Verification items for the finished model (mm, model axes). Coordinates: 2 decimals unless noted, no trailing zeros. Write each loop counter-clockwise with the first axis right and the second up, starting at its lowest first coordinate (ties: lowest second). Pieces come first, ordered by that corner, then holes. Notation, with made-up numbers: (-26.75, 47.5) - (16.25, 47.5) arc R8 cw to (16.25, 59.5) - close; hole circle Ø4 at (45.5, 61.5). An arc over 180 degrees is marked (long way). Answer as CSV lines item,"result". Start each with the question number.
```python
from build123d import *

# Parameters (mm, degrees)
ESBO_O1_W                = 103
ESBO_O1_H                = 55
RESSALTO_EXTRUS_O1_DEPTH = 3
ESBO_O2_W                = 3
ESBO_O2_H                = 15
CORTE_EXTRUS_O1_DEPTH    = 59.459387612
ESBO_O3_W                = 37
ESBO_O3_H                = 3
CORTE_EXTRUS_O2_DEPTH    = 59.459387612
ESBO_O4_W                = 97
ESBO_O4_H                = 10
CORTE_EXTRUS_O3_DEPTH    = 10
ESBO_O5_R                = 7.75
CORTE_EXTRUS_O4_DEPTH    = 59.459387612
CORTE_EXTRUS_O5_DEPTH    = 59.459387612
ESBO_O10_R               = 1
CORTE_EXTRUS_O6_DEPTH    = 59.459387612


with BuildPart() as part:
    # Esboço1 → Ressalto-extrusão1 (new body)
    with BuildSketch(Plane.XY):
        Rectangle(ESBO_O1_W, ESBO_O1_H)
    extrude(amount=RESSALTO_EXTRUS_O1_DEPTH)

    # Esboço2 → Corte-extrusão1 (cut, through all)
    with BuildSketch(Plane(origin=(0, 0, 0), x_dir=(-1, 0, 0), z_dir=(0, 0, -1))):
        with Locations((-50, 20)):
            Rectangle(ESBO_O2_W, ESBO_O2_H)
        with Locations((-50, -20)):
            Rectangle(ESBO_O2_W, ESBO_O2_H)
        with Locations((50, 20)):
            Rectangle(ESBO_O2_W, ESBO_O2_H)
        with Locations((50, -20)):
            Rectangle(ESBO_O2_W, ESBO_O2_H)
    extrude(amount=-CORTE_EXTRUS_O1_DEPTH, mode=Mode.SUBTRACT)

    # Esboço3 → Corte-extrusão2 (cut, through all)
    with BuildSketch(Plane(origin=(0, 0, 0), x_dir=(-1, 0, 0), z_dir=(0, 0, -1))):
        with Locations((0, -26)):
            Rectangle(ESBO_O3_W, ESBO_O3_H)
    extrude(amount=-CORTE_EXTRUS_O2_DEPTH, mode=Mode.SUBTRACT)

    # Esboço4 → Corte-extrusão3 (cut)
    with BuildSketch(Plane(origin=(0, 0, 0), x_dir=(-1, 0, 0), z_dir=(0, 0, -1))):
        with Locations((0, 22.5)):
            Rectangle(ESBO_O4_W, ESBO_O4_H)
    extrude(amount=-CORTE_EXTRUS_O3_DEPTH, mode=Mode.SUBTRACT)

    # Esboço5 → Corte-extrusão4 (cut, through all)
    with BuildSketch(Plane.XY.offset(3)):
        with Locations((-12.94, 1.5)):
            Circle(ESBO_O5_R)
        with Locations((12.94, 1.5)):
            Circle(ESBO_O5_R)
    extrude(amount=-CORTE_EXTRUS_O4_DEPTH, mode=Mode.SUBTRACT)

    # Esboço6 → Corte-extrusão5 (cut, through all)
    with BuildSketch(Plane(origin=(0, 0, 0), x_dir=(-1, 0, 0), z_dir=(0, 0, -1))):
        with BuildLine():
            Line((-9, -18.5), (9, -18.5))
            ThreePointArc((9, -18.5), (11.5, -16), (9, -13.5))
            Line((9, -13.5), (-9, -13.5))
            ThreePointArc((-9, -13.5), (-11.5, -16), (-9, -18.5))
        make_face()
    extrude(amount=-CORTE_EXTRUS_O5_DEPTH, mode=Mode.SUBTRACT)

    # Esboço10 → Corte-extrusão6 (cut, through all)
    with BuildSketch(Plane(origin=(0, 0, 0), x_dir=(-1, 0, 0), z_dir=(0, 0, -1))):
        with Locations((-21.285, 10.29)):
            Circle(ESBO_O10_R)
        with Locations((-21.285, -7.29)):
            Circle(ESBO_O10_R)
        with Locations((21.285, -7.29)):
            Circle(ESBO_O10_R)
        with Locations((21.285, 10.29)):
            Circle(ESBO_O10_R)
    extrude(amount=-CORTE_EXTRUS_O6_DEPTH, mode=Mode.SUBTRACT)


solid = part.part
```
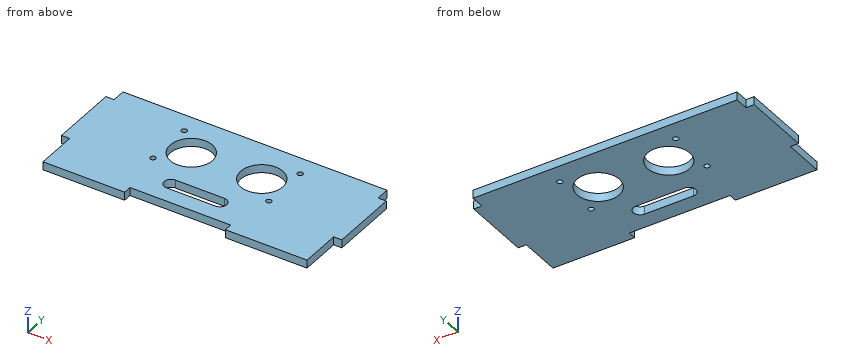
1. Scan lines: line 1 along Y through (x, z) = (-21.5, 0.4); line 2 along Y through (x, z) = (12.94, 1.55); line 3 along Y through (x, z) = (2, 0.45). Record each from-to range of solid material in increasing order. Write a range as from..to.
2. Cross-section at B-B (z = 2.15). Record the cut outline in (x, y) (3 decimals).
3. Cross-section at A-A (y = 1.5). Record the cut outline in (x, z), and give its area (3 significant figures).
4. Depth check by flat-ended pin: P1, Ø1.5, axis at y = -26.5, z = 1, coming from the +X side; P2, Ø0.9, axis at x = -50, z = 2, coming from the +Y side; P3, Ø1.5, axis at x = 49.5, z = 1, coming from the -Y side. Enter the tip coordinate at first touch or a pass-through.
5. Cross-section at D-D (y = 10.29). Record the cut outline in (x, z) (3 decimals).
6. Cross-section at C-C (x = 12.94). Record the cut outline in (y, z).
Completed:
1,line 1,"y = -27.5..-8.27, -6.31..9.31, 11.27..17.5"
1,line 2,"y = -24.5..-6.25, 9.25..17.5"
1,line 3,"y = -24.5..-18.5, -13.5..17.5"
2,outline,"(-51.5, -12.5) - (-48.5, -12.5) - (-48.5, -27.5) - (-18.5, -27.5) - (-18.5, -24.5) - (18.5, -24.5) - (18.5, -27.5) - (48.5, -27.5) - (48.5, -12.5) - (51.5, -12.5) - (51.5, 12.5) - (48.5, 12.5) - (48.5, 17.5) - (-48.5, 17.5) - (-48.5, 12.5) - (-51.5, 12.5) - close; hole circle Ø2 at (-21.285, -7.29); hole circle Ø2 at (-21.285, 10.29); hole circle Ø15.5 at (-12.94, 1.5); hole (-9, -18.5) - (9, -18.5) arc R2.5 ccw to (9, -13.5) - (-9, -13.5) arc R2.5 ccw to start; hole circle Ø15.5 at (12.94, 1.5); hole circle Ø2 at (21.285, -7.29); hole circle Ø2 at (21.285, 10.29)"
3,outline,"(-51.5, 0) - (-20.69, 0) - (-20.69, 3) - (-51.5, 3) - close; (-5.19, 0) - (5.19, 0) - (5.19, 3) - (-5.19, 3) - close; (20.69, 0) - (51.5, 0) - (51.5, 3) - (20.69, 3) - close"
3,area,"216 mm2"
4,P1,"stops at x = 48.5"
4,P2,"stops at y = 12.5"
4,P3,"stops at y = -12.5"
5,outline,"(-51.5, 0) - (-22.285, 0) - (-22.285, 3) - (-51.5, 3) - close; (-20.285, 0) - (20.285, 0) - (20.285, 3) - (-20.285, 3) - close; (22.285, 0) - (51.5, 0) - (51.5, 3) - (22.285, 3) - close"
6,outline,"(-24.5, 0) - (-6.25, 0) - (-6.25, 3) - (-24.5, 3) - close; (9.25, 0) - (17.5, 0) - (17.5, 3) - (9.25, 3) - close"
